Work out the finished part from the listing and answer in its coordinate system (mm). A direction names the side the tool comes from. Coordinates: 2 decimals unless noted, no trailing zeros. Write each loop counter-clockwise with the first axis right and the second up, starting at its lowest first coordinate (ties: lowest second). Pieces come first, ordered by that corner, then holes. Notation, with made-up numbers: M 78.5,9 L 82.5,9 A19 cw 82.5,17 Z; hole C 81,43.5 d11. An arc over 180 degrees is marked long. Use CSV: the item, a comma, the result in double quotes.
from build123d import *

# Parameters (mm, degrees)
SKETCH3_W           = 10
SKETCH3_H           = 10
SKETCH3_R           = 1.75
BOSS_EXTRUDE4_DEPTH = 11.5
CUT_EXTRUDE1_START  = 11.5
CUT_EXTRUDE1_DEPTH  = 5
SKETCH4_R           = 12.5
BOSS_EXTRUDE5_DEPTH = 1.5
SKETCH5_W           = 5
SKETCH5_H           = 5.8
CUT_EXTRUDE2_DEPTH  = 14.634995112
SKETCH6_R           = 6
BOSS_EXTRUDE6_DEPTH = 3
FILLET1_R           = 0.5
FILLET2_R           = 0.5
BOSS_EXTRUDE7_DEPTH = 5
FILLET3_R           = 0.5


with BuildPart() as part:
    # Sketch3 → Boss-Extrude4 (new body)
    with BuildSketch(Plane.XY):
        Rectangle(SKETCH3_W, SKETCH3_H)
        Circle(SKETCH3_R, mode=Mode.SUBTRACT)
    extrude(amount=BOSS_EXTRUDE4_DEPTH)

    # Sketch3<3> → Cut-Extrude1 (cut)
    with BuildSketch(Plane.XY.offset(CUT_EXTRUDE1_START)):
        Polygon((3.234529708, 0.866689623), (0.866689623, 3.234529708), (-2.367840085, 2.367840085), (-3.234529708, -0.866689623), (-0.866689623, -3.234529708), (2.367840085, -2.367840085), align=None)
    extrude(amount=-CUT_EXTRUDE1_DEPTH, mode=Mode.SUBTRACT)

    # Sketch4 → Boss-Extrude5 (add)
    with BuildSketch(Plane.XY.offset(11.5)):
        Circle(SKETCH4_R)
        Polygon((3.234529708, 0.866689623), (0.866689623, 3.234529708), (-2.367840085, 2.367840085), (-3.234529708, -0.866689623), (-0.866689623, -3.234529708), (2.367840085, -2.367840085), align=None, mode=Mode.SUBTRACT)
    extrude(amount=BOSS_EXTRUDE5_DEPTH)

    # Sketch5 → Cut-Extrude2 (cut, through all)
    with BuildSketch(Plane(origin=(2.92867424, -4.460901648, 0), x_dir=(0, 0, 1), z_dir=(0.965925826, 0.258819045, 0))):
        with Locations((9, -5.066896781)):
            Rectangle(SKETCH5_W, SKETCH5_H)
    extrude(amount=CUT_EXTRUDE2_DEPTH, mode=Mode.SUBTRACT)

    # Sketch6 → Boss-Extrude6 (add)
    with BuildSketch(Plane.XY.offset(13)):
        Circle(SKETCH6_R)
    extrude(amount=BOSS_EXTRUDE6_DEPTH)

    # Fillet1
    fillet1_edges = [part.edges().sort_by_distance(p)[0] for p in [
        (-0.750575231, 2.801184896, 13),
        (-2.801184896, 0.750575231, 13),
        (-2.050609665, -2.050609665, 13),
        (0.750575231, -2.801184896, 13),
    ]]
    fillet(fillet1_edges, radius=FILLET1_R)

    # Fillet2
    fillet2_edges = [part.edges().sort_by_distance(p)[0] for p in [
        (-6, 0, 13),
    ]]
    fillet(fillet2_edges, radius=FILLET2_R)

    # Sketch7 → Boss-Extrude7 (add)
    with BuildSketch(Plane.XY.offset(16)):
        with BuildLine():
            Line((-1.833030278, -0.8), (1.833030278, -0.8))
            ThreePointArc((1.833030278, -0.8), (0, 2), (-1.833030278, -0.8))
        make_face()
    extrude(amount=BOSS_EXTRUDE7_DEPTH)

    # Fillet3
    fillet3_edges = [part.edges().sort_by_distance(p)[0] for p in [
        (0, 2, 16),
        (0, -0.8, 16),
    ]]
    fillet(fillet3_edges, radius=FILLET3_R)


solid = part.part
Item 1: Consider probe 1 along X at (y, z) = (0, 4.25); probe 2 along Z at (x, y) = (5.5, -4.25). Determine where each line is inside the solid, lowest interval first.
Answer:
probe 1,"x = -5 to -1.75, 1.75 to 5"
probe 2,"z = 11.5 to 13"
Item 2: Given pin 1 (11 mm diameter, centred on x = -0.5, z = 7, fed in from +Y); pin 2 (1.5 mm diameter, centred on x = 2.5, z = 13, fed in from +Y); pin 3 (8 mm diameter, centred on y = 8.5, z = 12, fed in from +X); pin 4 (5 mm diameter, centred on y = -4, z = 4, fed in from +X), each flat-ended and moving along its own axis, determine where each tip first touches the part or whether it passes through.
Answer:
pin 1,"stops at y = 12.5"
pin 2,"stops at y = 12.38"
pin 3,"stops at x = 11.66"
pin 4,"stops at x = 5"
Item 3: For a pull along X with two mould halves and no side action, classify faces 6 (the face through (11.923, 3.755, 12.24)), 7 (the face through (2, 0, 0)), 8 (the face through (-2.66, 0.69, 12.86)) as released by +X, released by -X, zero draft, split by the parting line, or undercut.
Answer:
face 6,"split by the parting line"
face 7,"zero draft"
face 8,"undercut"
Item 4: A tool of negligible diameter and unlimited length cuts with its end or side. For faces 1 (the face through (1.617, -0.67, 3.204)), 2 (the face through (5, -5, 13)), 3 (the face through (0, -0.8, 19)), 4 (the face through (-0.599, 2.694, 12.85)), 5 (the face through (-5, 0, 6)), from which of +Z, -Z, +X, -X, +Y, -Y can it reach the whole face along a straight path? Write none if from no direction.
Answer:
face 1,"-Z"
face 2,"+Z"
face 3,"+Z, +X, -X, -Y"
face 4,"none"
face 5,"-Z, -X, +Y, -Y"
Item 5: The part is cut by section C-C (x = -7.5). Write down the section's boundary in (y, z), then the cut area to 3 significant figures.
Answer:
outline,"M -10,11.5 L 10,11.5 L 10,13 L -10,13 Z"
area,"30.0 mm2"
Item 6: The part is cut by section B-B (z = 3.5). Write down the section's boundary in (x, y), then the cut area to 3 significant figures.
Answer:
outline,"M -5,-5 L 5,-5 L 5,5 L -5,5 Z; hole C 0,0 d3.5"
area,"90.4 mm2"
Item 7: The part is cut by section A-A (z = 9.75). Write down the section's boundary in (x, y).
Answer:
outline,"M -5,-5 L 5,-5 L 5,-1.66 L -0.87,-3.23 L -3.23,-0.87 L -2.37,2.37 L 5,4.34 L 5,5 L -5,5 Z"
